The model under review builds one solid part; all positions refer to its coordinate system, in mm. Face numbers are marked on the shaded views. A direction names the side the tool comes from. Give positions to 0.01 mm unless a question says otherwise; leave off trailing zeros. Loops run counter-clockwise (first coordinate to the right, second up) from the corner with the lowest first, then second, coordinate; pieces in that order, holes last. Notation, with made-up numbers: (57.25, -8.5) - (69.25, -8.5) arc R24 ccw to (69.25, 8.5) - close; hole circle Ø9 at (50, 15). An arc over 180 degrees is marked (long way). Answer as a JSON object with one key per item and string values.
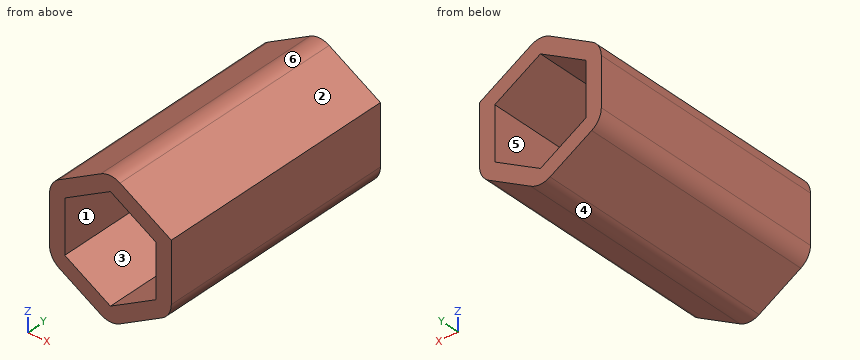
Autodesk Inventor part; units mm, degrees
ref_plane "YZ Plane" through (0, 0, 0) normal (1, 0, 0) x (0, 1, 0)
ref_plane "XZ Plane" through (0, 0, 0) normal (0, 1, 0) x (-1, 0, 0)
ref_plane "XY Plane" through (0, 0, 0) normal (0, 0, 1) x (1, 0, 0)
sketch "Sketch1" plane through (0, 0, 0) normal (0, 1, 0) x (-1, 0, 0)
  line L0 (0, 0) -> (6.35, -3.6662)
  line L1 (6.35, -3.6662) -> (6.35, -10.9985)
  line L2 (6.35, -10.9985) -> (0, -14.6647)
  line L3 (0, -14.6647) -> (-6.35, -10.9985)
  line L4 (-6.35, -10.9985) -> (-6.35, -3.6662)
  line L5 (-6.35, -3.6662) -> (0, 0)
  line L6 (0, 0) -> (0, -14.6647) construction
  line L7 (6.35, -10.9985) -> (-6.35, -3.6662) construction
  line L8 (6.35, -3.6662) -> (-6.35, -10.9985) construction
  line L9 (0, -1.8331) -> (4.7625, -4.5827)
  line L10 (4.7625, -4.5827) -> (4.7625, -10.082)
  line L11 (4.7625, -10.082) -> (0, -12.8316)
  line L12 (0, -12.8316) -> (-4.7625, -10.082)
  line L13 (-4.7625, -10.082) -> (-4.7625, -4.5827)
  line L14 (-4.7625, -4.5827) -> (0, -1.8331)
  line L15 (4.7625, -4.5827) -> (-4.7625, -10.082) construction
  line L16 (0, -12.8316) -> (0, -1.8331) construction
  line L17 (4.7625, -10.082) -> (-4.7625, -4.5827) construction
  point P0 (0, -7.3323)
  dimension "d0" = 12.7
  dimension "d2" = 9.525
extrude "Extrusion1" add sketch "Sketch1" along normal blind 25.4
fillet "Fillet1" radius 2 5 edges at (0, 12.7, 0) (-6.35, 12.7, -3.6662) (-6.35, 12.7, -10.9985) (0, 12.7, -14.6647) (6.35, 12.7, -10.9985)
properties part number "arm wheel spacer"
Q1. For the marked faces 5 and 6, list the 3-axis set-ups (+Z, -Z, +X, -X, +Y, -Y) from which the entire face can be reached by the end or side of a thin tool; tool diameter is ignored.
Results:
{"face 5": "+Y, -Y", "face 6": "+Z, +Y, -Y"}
Q2. Consider section C-C, the plane x = 4. State the section outline as (y, z) points.
Results:
{"outline": "(0, -12.36) - (25.4, -12.36) - (25.4, -10.52) - (0, -10.52) - close; (0, -4.14) - (25.4, -4.14) - (25.4, -2.31) - (0, -2.31) - close"}
Q3. Consider section B-B, the plane y = 12.5. State the section outline as (x, z) points.
Results:
{"outline": "(-6.35, -9.84) arc R2 ccw to (-5.35, -11.58) - (-1, -14.09) arc R2 ccw to (1, -14.09) - (5.35, -11.58) arc R2 ccw to (6.35, -9.84) - (6.35, -3.67) - (1, -0.58) arc R2 ccw to (-1, -0.58) - (-5.35, -3.09) arc R2 ccw to (-6.35, -4.82) - close; hole (-4.76, -10.08) - (0, -12.83) - (4.76, -10.08) - (4.76, -4.58) - (0, -1.83) - (-4.76, -4.58) - close"}
Q4. Consider section D-D, the plane z = -1. State the section outline as (x, y) points, plus the area to 3 significant figures.
Results:
{"outline": "(-1.73, 0) - (1.73, 0) - (1.73, 25.4) - (-1.73, 25.4) - close", "area": "88.0 mm^2"}
Q5. The part is to be moulded in two halves that separate along X. For the marked faces 1, 2, 3 and 4, say which applies: +X half, -X half, draft (parallel to the pull), parting line (faces both ways), or undercut.
Results:
{"face 1": "undercut", "face 2": "+X half", "face 3": "undercut", "face 4": "parting line"}
Q6. Clearance check with flat-ended pins moving along their axes: pin 1 Ø1 at (x, y) = (1, 8.5) entering from +Z; pin 2 Ø1.5 at (x, z) = (5, -13) entering from -Y. State where each tip first meets the part, or that it passes through.
Results:
{"pin 1": "stops at z = -0.37", "pin 2": "passes through"}
Q7. To check wall thickness, follow probe 1 along X at (y, z) = (6.5, -10); probe 2 along X at (y, z) = (8.75, -9.25); probe 3 along Z at (x, y) = (4.5, 22.5). State the ranges of each line that lie inside material, in increasing order. Write a range as [from, to].
Results:
{"probe 1": "x = [-6.34, -4.76], [4.76, 6.34]", "probe 2": "x = [-6.35, -4.76], [4.76, 6.35]", "probe 3": "z = [-12.07, -10.23], [-4.43, -2.6]"}
Q8. Consider section A-A, the plane z = -5.5. State the section outline as (x, y) points, plus the area to 3 significant figures.
Results:
{"outline": "(-6.35, 0) - (-4.76, 0) - (-4.76, 25.4) - (-6.35, 25.4) - close; (4.76, 0) - (6.35, 0) - (6.35, 25.4) - (4.76, 25.4) - close", "area": "80.6 mm^2"}
